For this review, take the finished solid that the model builds, in its own axes (mm). Coordinates: 2 decimals unless noted, no trailing zeros.
1. Take a section at A-A, the plane z = -237.5. Count the separate pieces of the cut face and the enclosed holes in it, then the cut area to 3 significant figures.
2. To check wall thickness, follow probe 1 along Y at (x, z) = (20.5, 39.5); probe 2 along Y at (x, z) = (30, -31.5); probe 3 along X at (y, z) = (-8.5, -102). State the ranges of each line that lie inside material, in increasing order.
3. Clearance check with flat-ended pins moving along their axes: P1, Ø6, axis at x = -10.5, z = -46, coming from the +Y side; P2, Ø1, axis at x = -9, z = -89, coming from the +Y side; P3, Ø5, axis at y = 0.5, z = -36, coming from the -X side. State where each tip first meets the part, or that it passes through.
```python
from build123d import *

# Parameters (mm, degrees)
SKETCH1_R      = 2.1
EXTRUDE1_DEPTH = 284.8


with BuildPart() as part:
    # Sketch1 → Extrude1 (new, symmetric)
    with BuildSketch(Plane.XY):
        with BuildLine():
            Line((-38.199999929, 10), (-34.639999675, 10))
            Line((-34.639999675, 10), (-32.839999603, 8.2))
            Line((-32.839999603, 8.2), (-35.499339671, 8.2))
            Line((-35.499339671, 8.2), (-35.499339671, 6.56))
            Line((-35.499339671, 6.56), (-32.839999603, 3.900660038))
            Line((-32.839999603, 3.900660038), (-27.159999603, 3.900660038))
            Line((-27.159999603, 3.900660038), (-24.500659536, 6.56))
            Line((-24.500659536, 6.56), (-24.500659536, 8.2))
            Line((-24.500659536, 8.2), (-27.159999603, 8.2))
            Line((-27.159999603, 8.2), (-25.359999532, 10))
            Line((-25.359999532, 10), (-14.640000468, 10))
            Line((-14.640000468, 10), (-12.840000397, 8.2))
            Line((-12.840000397, 8.2), (-15.499340464, 8.2))
            Line((-15.499340464, 8.2), (-15.499340464, 6.56))
            Line((-15.499340464, 6.56), (-12.840000397, 3.900660038))
            Line((-12.840000397, 3.900660038), (-7.159998809, 3.900660038))
            Line((-7.159998809, 3.900660038), (-4.500658742, 6.56))
            Line((-4.500658742, 6.56), (-4.500658742, 8.2))
            Line((-4.500658742, 8.2), (-7.159998809, 8.2))
            Line((-7.159998809, 8.2), (-5.359998738, 10))
            Line((-5.359998738, 10), (5.359998738, 10))
            Line((5.359998738, 10), (7.159998809, 8.2))
            Line((7.159998809, 8.2), (4.500658742, 8.2))
            Line((4.500658742, 8.2), (4.500658742, 6.56))
            Line((4.500658742, 6.56), (7.159998809, 3.900660038))
            Line((7.159998809, 3.900660038), (12.840000397, 3.900660038))
            Line((12.840000397, 3.900660038), (15.499340464, 6.56))
            Line((15.499340464, 6.56), (15.499340464, 8.2))
            Line((15.499340464, 8.2), (12.840000397, 8.2))
            Line((12.840000397, 8.2), (14.640000468, 10))
            Line((14.640000468, 10), (25.359999532, 10))
            Line((25.359999532, 10), (27.159999603, 8.2))
            Line((27.159999603, 8.2), (24.500659536, 8.2))
            Line((24.500659536, 8.2), (24.500659536, 6.56))
            Line((24.500659536, 6.56), (27.159999603, 3.900660038))
            Line((27.159999603, 3.900660038), (32.839999603, 3.900660038))
            Line((32.839999603, 3.900660038), (35.499339671, 6.56))
            Line((35.499339671, 6.56), (35.499339671, 8.2))
            Line((35.499339671, 8.2), (32.839999603, 8.2))
            Line((32.839999603, 8.2), (34.639999675, 10))
            Line((34.639999675, 10), (38.199999929, 10))
            ThreePointArc((38.199999929, 10), (39.47279216, 9.472792181), (39.999999929, 8.199999929))
            Line((39.999999929, 8.199999929), (39.999999787, 4.639999675))
            Line((39.999999787, 4.639999675), (38.199999716, 2.839999675))
            Line((38.199999716, 2.839999675), (38.199999821, 5.499339742))
            Line((38.199999821, 5.499339742), (36.559999821, 5.499339807))
            Line((36.559999821, 5.499339807), (33.900659754, 2.839999845))
            Line((33.900659754, 2.839999845), (33.900659641, 0))
            Line((33.900659641, 0), (33.900659754, -2.839999845))
            Line((33.900659754, -2.839999845), (36.559999821, -5.499339807))
            Line((36.559999821, -5.499339807), (38.199999821, -5.499339742))
            Line((38.199999821, -5.499339742), (38.199999716, -2.839999675))
            Line((38.199999716, -2.839999675), (39.999999787, -4.639999675))
            Line((39.999999787, -4.639999675), (39.999999929, -8.199999929))
            ThreePointArc((39.999999929, -8.199999929), (39.47279216, -9.472792181), (38.199999929, -10))
            Line((38.199999929, -10), (34.639999675, -10))
            Line((34.639999675, -10), (32.839999603, -8.2))
            Line((32.839999603, -8.2), (35.499339671, -8.2))
            Line((35.499339671, -8.2), (35.499339671, -6.56))
            Line((35.499339671, -6.56), (32.839999603, -3.900660038))
            Line((32.839999603, -3.900660038), (27.159999603, -3.900660038))
            Line((27.159999603, -3.900660038), (24.500659536, -6.56))
            Line((24.500659536, -6.56), (24.500659536, -8.2))
            Line((24.500659536, -8.2), (27.159999603, -8.2))
            Line((27.159999603, -8.2), (25.359999532, -10))
            Line((25.359999532, -10), (14.640000468, -10))
            Line((14.640000468, -10), (12.840000397, -8.2))
            Line((12.840000397, -8.2), (15.499340464, -8.2))
            Line((15.499340464, -8.2), (15.499340464, -6.56))
            Line((15.499340464, -6.56), (12.840000397, -3.900660038))
            Line((12.840000397, -3.900660038), (7.159998809, -3.900660038))
            Line((7.159998809, -3.900660038), (4.500658742, -6.56))
            Line((4.500658742, -6.56), (4.500658742, -8.2))
            Line((4.500658742, -8.2), (7.159998809, -8.2))
            Line((7.159998809, -8.2), (5.359998738, -10))
            Line((5.359998738, -10), (-5.359998738, -10))
            Line((-5.359998738, -10), (-7.159998809, -8.2))
            Line((-7.159998809, -8.2), (-4.500658742, -8.2))
            Line((-4.500658742, -8.2), (-4.500658742, -6.56))
            Line((-4.500658742, -6.56), (-7.159998809, -3.900660038))
            Line((-7.159998809, -3.900660038), (-12.840000397, -3.900660038))
            Line((-12.840000397, -3.900660038), (-15.499340464, -6.56))
            Line((-15.499340464, -6.56), (-15.499340464, -8.2))
            Line((-15.499340464, -8.2), (-12.840000397, -8.2))
            Line((-12.840000397, -8.2), (-14.640000468, -10))
            Line((-14.640000468, -10), (-25.359999532, -10))
            Line((-25.359999532, -10), (-27.159999603, -8.2))
            Line((-27.159999603, -8.2), (-24.500659536, -8.2))
            Line((-24.500659536, -8.2), (-24.500659536, -6.56))
            Line((-24.500659536, -6.56), (-27.159999603, -3.900660038))
            Line((-27.159999603, -3.900660038), (-32.839999603, -3.900660038))
            Line((-32.839999603, -3.900660038), (-35.499339671, -6.56))
            Line((-35.499339671, -6.56), (-35.499339671, -8.2))
            Line((-35.499339671, -8.2), (-32.839999603, -8.2))
            Line((-32.839999603, -8.2), (-34.639999675, -10))
            Line((-34.639999675, -10), (-38.199999929, -10))
            ThreePointArc((-38.199999929, -10), (-39.47279216, -9.472792181), (-39.999999929, -8.199999929))
            Line((-39.999999929, -8.199999929), (-39.999999787, -4.639999675))
            Line((-39.999999787, -4.639999675), (-38.199999716, -2.839999675))
            Line((-38.199999716, -2.839999675), (-38.199999821, -5.499339742))
            Line((-38.199999821, -5.499339742), (-36.559999821, -5.499339807))
            Line((-36.559999821, -5.499339807), (-33.900659754, -2.839999845))
            Line((-33.900659754, -2.839999845), (-33.900659641, 0))
            Line((-33.900659641, 0), (-33.900659754, 2.839999845))
            Line((-33.900659754, 2.839999845), (-36.559999821, 5.499339807))
            Line((-36.559999821, 5.499339807), (-38.199999821, 5.499339742))
            Line((-38.199999821, 5.499339742), (-38.199999716, 2.839999675))
            Line((-38.199999716, 2.839999675), (-39.999999787, 4.639999675))
            Line((-39.999999787, 4.639999675), (-39.999999929, 8.199999929))
            ThreePointArc((-39.999999929, 8.199999929), (-39.47279216, 9.472792181), (-38.199999929, 10))
        make_face()
        with Locations((-29.999999603, 0)):
            Circle(SKETCH1_R, mode=Mode.SUBTRACT)
        with Locations((-9.999999603, 0)):
            Circle(SKETCH1_R, mode=Mode.SUBTRACT)
        with Locations(Location((29.999999603, 0, 0), (0, 0, 180))):
            Circle(SKETCH1_R, mode=Mode.SUBTRACT)
        with Locations(Location((9.999999603, 0, 0), (0, 0, 180))):
            Circle(SKETCH1_R, mode=Mode.SUBTRACT)
        Polygon((-38.199999929, 8.2), (-38.199999864, 6.569339742), (-37.629999799, 6.569339742), (-36.569339648, 7.629999935), (-36.569339648, 8.2), align=None, mode=Mode.SUBTRACT)
        Polygon((-17.3, 6.239339079), (-17.3, 8.2), (-22.7, 8.2), (-22.7, 6.239339079), (-26.099339368, 2.839999845), (-26.099339368, -2.839999845), (-22.7, -6.239339079), (-22.7, -8.2), (-17.3, -8.2), (-17.3, -6.239339079), (-13.900660632, -2.839999845), (-13.900660632, 2.839999845), align=None, mode=Mode.SUBTRACT)
        Polygon((-6.099339678, -2.840000949), (-6.099339678, 2.840000949), (-2.700001413, 6.239339079), (-2.700001413, 8.2), (2.700001413, 8.2), (2.700001413, 6.239339079), (6.099339678, 2.840000949), (6.099339678, -2.840000949), (2.700001413, -6.239339079), (2.700001413, -8.2), (-2.700001413, -8.2), (-2.700001413, -6.239339079), align=None, mode=Mode.SUBTRACT)
        Polygon((-36.569339648, -7.629999935), (-36.569339648, -8.2), (-38.199999929, -8.2), (-38.199999864, -6.569339742), (-37.629999799, -6.569339742), align=None, mode=Mode.SUBTRACT)
        Polygon((36.569339648, 8.2), (38.199999929, 8.2), (38.199999864, 6.569339742), (37.629999799, 6.569339742), (36.569339648, 7.629999935), align=None, mode=Mode.SUBTRACT)
        Polygon((36.569339648, -8.2), (38.199999929, -8.2), (38.199999864, -6.569339742), (37.629999799, -6.569339742), (36.569339648, -7.629999935), align=None, mode=Mode.SUBTRACT)
        Polygon((13.900660632, -2.839999845), (17.3, -6.239339079), (17.3, -8.2), (22.7, -8.2), (22.7, -6.239339079), (26.099339368, -2.839999845), (26.099339368, 2.839999845), (22.7, 6.239339079), (22.7, 8.2), (17.3, 8.2), (17.3, 6.239339079), (13.900660632, 2.839999845), align=None, mode=Mode.SUBTRACT)
    extrude(amount=EXTRUDE1_DEPTH, both=True)


solid = part.part
```
Results list:
1. separate pieces: 1
1. enclosed holes: 11
1. area: 546 mm2
2. probe 1: y = -10 to -8.2, 8.2 to 10
2. probe 2: y = -3.9 to -2.1, 2.1 to 3.9
2. probe 3: x = -39.97 to -33.14, -26.86 to -13.14, -6.86 to 6.86, 13.14 to 26.86, 33.14 to 39.97
3. P1: stops at y = 8.86
3. P2: stops at y = 3.9
3. P3: stops at x = -38.36
